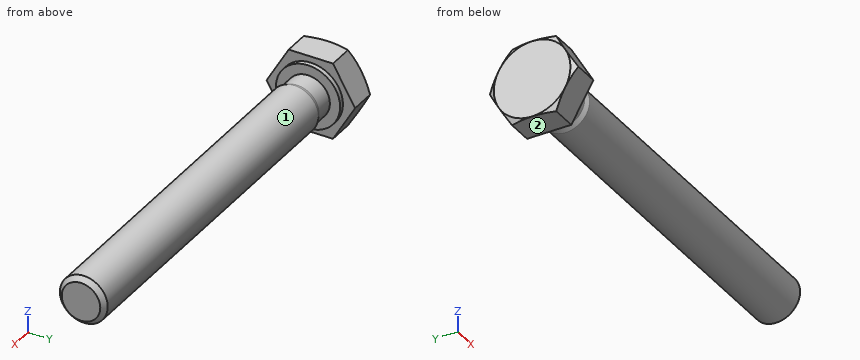
Autodesk Inventor part; units mm, degrees
ref_plane "Work Plane1" through (1.525, 0, 0) normal (0, 0, 1) x (1, 0, 0)
ref_plane "YZ Plane" through (0, 0, 0) normal (1, 0, 0) x (0, 1, 0)
ref_plane "XZ Plane" through (0, 0, 0) normal (0, 1, 0) x (-1, 0, 0)
sketch "Sketch1" plane through (0, 0, 0) normal (0, 0, 1) x (1, 0, 0)
  line L0 (0, 3.35) -> (0, 2.2835)
  line L1 (2.4, 2.5) -> (40, 2.5)
  line L2 (40, 2.5) -> (40, 0)
  line L3 (40, 0) -> (-0.5001, 0)
  line L4 (-8.6001, 0) -> (48.1, 0)
  line L5 (-0.5001, 0) -> (-0.5001, 3.35)
  line L6 (-0.5001, 3.35) -> (0, 3.35)
  line L7 (2.4, 2.5) -> (1.9091, 2.2835)
  line L8 (1.9091, 2.2835) -> (0, 2.2835)
  line L9 (0, -0.67) -> (0, 4.02)
  dimension "d0" = 40
  dimension "d1" = 37.6
  dimension "d2" = 5
  dimension "d9" = 0.5001
  dimension "d10" = 6.7
  dimension "d13" = 0.4909
  dimension "d14" = 4.567
revolve "Body" add sketch "Sketch1" angle 360 about axis through (40, 0, 0) along (-1, 0, 0)
sketch "Sketch2" plane through (-0.5001, 0, 0) normal (-1, 0, 0) x (0, 0, 1)
  line L0 (0, 4.6188) -> (4, 2.3094)
  line L1 (4, 2.3094) -> (4, -2.3094)
  line L2 (4, -2.3094) -> (0, -4.6188)
  line L3 (0, -4.6188) -> (-4, -2.3094)
  line L4 (-4, -2.3094) -> (-4, 2.3094)
  line L5 (-4, 2.3094) -> (0, 4.6188)
  point P0 (0, 0)
  point P1 (0, 0)
  dimension "d11" = 8
extrude "Head" add sketch "Sketch2" along normal blind 3
sketch "Sketch4" plane through (0, 0, 0) normal (0, 0, 1) x (1, 0, 0)
  line L0 (-3.5001, 4) -> (-3.5001, 4.6188)
  line L1 (-3.5001, 4.6188) -> (-3.1428, 4.6188)
  line L2 (-3.1428, 4.6188) -> (-3.5001, 4)
  line L3 (-4.1001, 0) -> (0.0999, 0)
  line L4 (-0.5001, 4.6188) -> (-3.5001, 4.6188)
  line L5 (-3.5001, 2.3094) -> (-3.5001, 4.6188)
  dimension "d5" = 30
  dimension "d19" = 8
revolve "Chamfer1" cut sketch "Sketch4" angle 360 about axis through (-10, 0, 0) along (1, 0, 0)
thread "Thread"
chamfer "Chamfer2" distance 0.4908 distance2 0.4909 1 edges at (40, -2.5, 0) measured on face at (40, 0.1004, 0.4284)
ref_plane "Work Plane1" through (1.525, 0, 0) normal (0, 0, 1) x (1, 0, 0)
equation "\"d0\" = NLG"
equation "\"d1\" = GEL"
equation "\"d2\" = GD"
equation "\"d10\" = SD2"
equation "\"d14\" = BDM"
equation "\"d11\" = SW"
equation "\"d3\" = KOH - SD"
equation "\"d5\" = ANG1"
equation "\"d19\" = SW0"
equation "\"d15\" = GEL"
equation "\"d6\" = -0.5 * SPD + 0.5 * GD"
equation "\"NLG\" = 40"
equation "\"GD\" = NND"
equation "\"BDM\" = 4.56699"
equation "\"KOH\" = 3.5"
equation "\"GEL\" = 37.6"
equation "\"SW\" = 8"
equation "\"SW0\" = 8"
equation "\"SPD\" = NND - 1.2269 * PTC"
equation "\"SD2\" = 6.7"
equation "\"SD\" = 0.5"
equation "\"ANG1\" = 30deg"
equation "\"GAL\" = 0.61345 * PTC"
equation "\"GUL\" = 0.61345 * PTC"
equation "\"RR\" = 0.2"
equation "\"GD1\" = THREADDIA - 1.2269 * PTC"
equation "\"THREADDIA\" = 5"
equation "\"TOA\" = 30deg"
equation "\"PTC\" = 0.8"
equation "\"NND\" = 5"
equation "\"E0\" = 1.155 * SW"
properties part number "DIN 933 - M5  x 40" material "Steel, Mild"
Geometry check sheet. Reference: the model listing, model coordinates, mm. Face numbers are marked on the shaded views. A direction names the side the tool comes from. Give positions to 0.01 mm unless a question says otherwise; leave off trailing zeros. Order: outer loops, then holes, each group sorted by start corner. A loop starts at its lowest first (then second) coordinate and runs counter-clockwise, first axis right, second up.
1. Depth check by flat-ended pin: pin 1 (5 mm diameter, centred on x = 16.5, y = 1, fed in from -Z); pin 2 (2 mm diameter, centred on x = 15.5, z = -2, fed in from +Y); pin 3 (3 mm diameter, centred on x = 14.5, z = -1, fed in from -Y). Enter the tip coordinate at first touch or a pass-through.
Completed:
pin 1: stops at z = -2.5
pin 2: stops at y = 2.29
pin 3: stops at y = -2.5
2. Scan lines: line 1 (X direction, y = 3, z = 2.5); line 2 (Y direction, x = 23.5, z = 0). Record each from-to range of solid material in increasing order.
Completed:
line 1: x = -3.5 to -0.5
line 2: y = -2.5 to 2.5
3. Sectioned sample at A-A (x = 7). Record the boundary of the cut face in (y, z).
Completed:
outline: circle Ø5 at (0, 0)
4. Access from +Z, -Z, +X, -X, +Y, -Y to the whole of each face (thin tool, end or side, straight path). Record for the marked faces 1 and 2.
Completed:
face 1: +X
face 2: -Z, +X, -X, +Y, -Y
